Part print with two shaded views. Sizes in mm from the minimum x, y, z corner. A direction names the side the tool comes from. Round coordinates to 2 decimals unless told otherwise and drop trailing zeros. Order: outer loops, then holes, each group sorted by start corner. A loop starts at its lowest first (then second) coordinate and runs counter-clockwise, first axis right, second up. Notation, with made-up numbers: (17, 58) - (24, 58) arc R23 cw to (24, 75) - close; hole circle Ø5 at (-19, 43). An arc over 180 degrees is marked (long way). Write item = value, one per line.
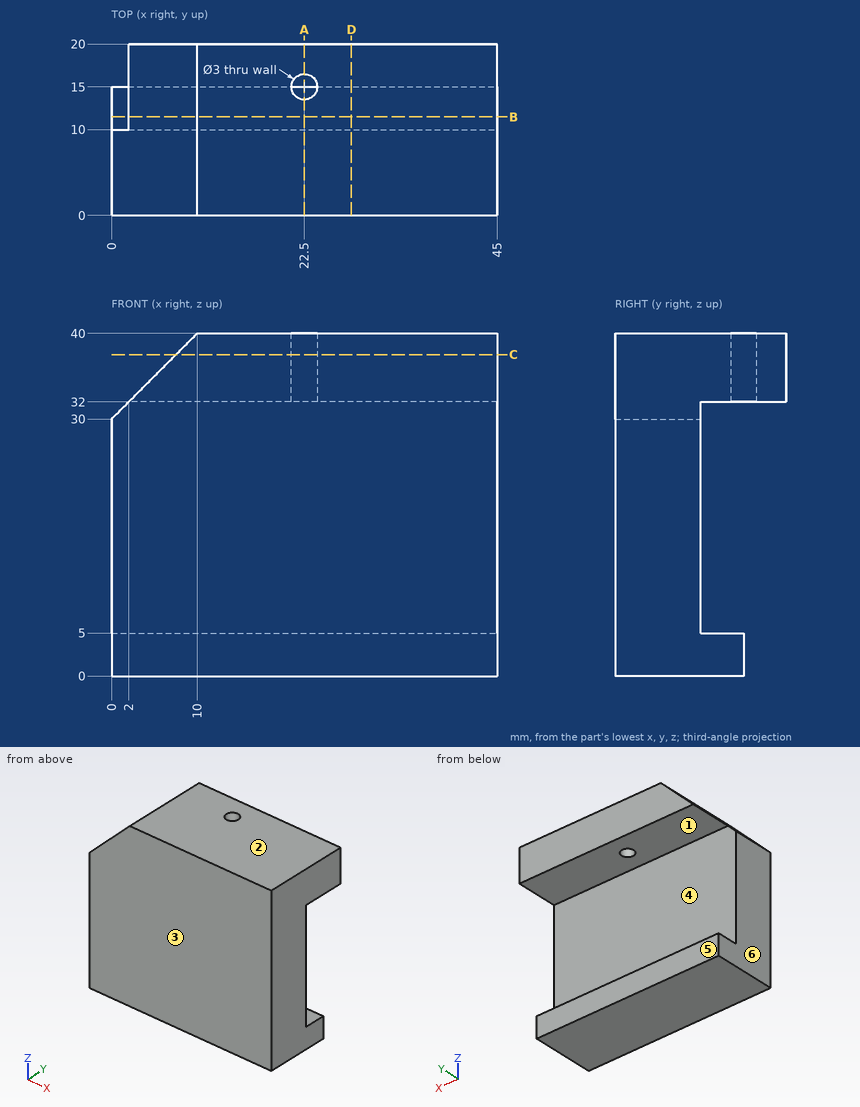
1) 3-axis set-ups, long thin cutter, end or side, ignore diameter. For the marked faces 5 and 6: which of +Z, -Z, +X, -X, +Y, -Y reach the whole face in a straight line?
Conclusion:
face_5 = -Z, +X, -X, +Y
face_6 = +Z, -Z, -X, +Y, -Y
2) Flat gauge pins, fed straight in: pin 1 Ø21.5 at (x, z) = (14.5, 19.5) entering from +Y; pin 2 Ø1.5 at (x, z) = (39, 6.5) entering from -Y; pin 3 Ø2.5 at (x, z) = (30.5, 3.5) entering from +Y; pin 4 Ø1.8 at (x, y) = (22.5, 15) entering from +Z. Where does each tip first touch, or does it go through?
Conclusion:
pin_1 = 10
pin_2 = 0
pin_3 = 15
pin_4 = 5
3) Cut at D-D (x = 28). Write the cut outline in (y, z), and give its area (3 significant figures).
Conclusion:
outline = (0, 0) - (15, 0) - (15, 5) - (10, 5) - (10, 32) - (20, 32) - (20, 40) - (0, 40) - close
area = 505 mm^2
4) Cut at B-B (y = 11.5). Write the cut outline in (x, z), and give its area (3 significant figures).
Conclusion:
outline = (0, 0) - (45, 0) - (45, 5) - (0, 5) - close; (2, 32) - (45, 32) - (45, 40) - (10, 40) - close
area = 537 mm^2
5) Mould opens along Z. For the marked faces 1, 2, 3 and 4 say: +Z half, -Z half, draft (parallel to the pull), parting line (faces both ways), or undercut.
Conclusion:
face_1 = undercut
face_2 = +Z half
face_3 = draft
face_4 = undercut
6) Cut at C-C (z = 37.5). Write the cut outline in (x, y).
Conclusion:
outline = (7.5, 0) - (45, 0) - (45, 20) - (7.5, 20) - close; hole circle Ø3 at (22.5, 15)
7) Cut at A-A (x = 22.5). Write the cut outline in (y, z).
Conclusion:
outline = (0, 0) - (15, 0) - (15, 5) - (10, 5) - (10, 32) - (13.5, 32) - (13.5, 40) - (0, 40) - close; (16.5, 32) - (20, 32) - (20, 40) - (16.5, 40) - close
8) Wall check: line 1 along Y through (x, z) = (22.5, 38); line 2 along Z through (x, y) = (31, 12); line 3 along Z through (x, y) = (19.5, 19). Give the ranges that are in metal, low to high.
Conclusion:
line_1 = 0 to 13.5, 16.5 to 20
line_2 = 0 to 5, 32 to 40
line_3 = 32 to 40
